Part model, mm, in its own coordinate system. Round coordinates to 2 decimals unless told otherwise and drop trailing zeros. Order: outer loops, then holes, each group sorted by start corner. A loop starts at its lowest first (then second) coordinate and runs counter-clockwise, first axis right, second up. Notation, with made-up numbers: M -15.75,-10.75 L 36.25,-10.75 A24 ccw 36.25,5.25 Z; hole C -40,48 d1. An arc over 180 degrees is marked long. Write each question's results on one line, items separated by ' | '. Start each with the question number.
1. Probe L1, parallel to Y at x = 1.15, z = -12.7; L2, parallel to Y at x = 2.05, z = -45; L3, parallel to Z at x = 2.3, y = -13.5. List the from-to ranges inside material, lowest first. Write a range as [from, to].
2. Drop a flat-ended pin along its axis: pin 1 Ø1.5 at (x, y) = (0.5, -61) entering from +Z. Give the stop position or say it passes through.
3. Band-saw the part on D-D, the plane z = -68.5. List the corners of the cut face in (x, y) (3 decimals).
4. Band-saw the part on A-A, the plane z = -50.8. List the corners of the cut face in (x, y) (3 decimals), then the cut area to 3 significant figures.
5. Band-saw the part on B-B, the plane x = 1.4. Give the number of separate pieces and of enclosed holes in the cut face, then the cut area to 3 significant figures.
6. Band-saw the part on C-C, the plane y = -12.7. List the corners of the cut face in (x, z) (3 decimals), then the cut area to 3 significant figures.
Autodesk Inventor part; units mm, degrees
ref_plane "YZ Plane" through (0, 0, 0) normal (1, 0, 0) x (0, 1, 0)
ref_plane "XZ Plane" through (0, 0, 0) normal (0, 1, 0) x (-1, 0, 0)
ref_plane "XY Plane" through (0, 0, 0) normal (0, 0, 1) x (1, 0, 0)
sketch "Sketch1" plane through (0, 0, 0) normal (1, 0, 0) x (0, 1, 0)
  line L0 (0, 0) -> (0, -101.6)
  line L1 (0, -101.6) -> (-52.8555, -156.4884)
  line L2 (-25.4, 2.4125) -> (-25.4, -91.3586)
  line L3 (-25.4, -91.3586) -> (-71.1516, -138.8699)
  line L4 (-52.8555, -156.4884) -> (-71.1516, -138.8699)
  line L5 (0, 0) -> (-25.4, 0)
  dimension "d0" = 101.6
  dimension "d1" = 25.4
  dimension "d2" = 25.4
  dimension "d3" = 76.2
  dimension "d4" = 136.081
extrude "Extrusion1" add sketch "Sketch1" along normal blind 3.175
sketch "Sketch2" plane through (0, 0, 0) normal (-1, 0, 0) x (0, 0, 1)
  circle A0 centre (-12.7, -12.7) radius 3.3734
  circle A1 centre (-31.75, -12.7) radius 3.3734
  circle A2 centre (-50.8, -12.7) radius 3.3734
  line L0 (0, -25.4) -> (0, 0)
  line L1 (0, -12.7) -> (-114.7885, -12.7) construction
  line L2 (-156.4884, -52.8555) -> (-101.6, 0)
  circle A3 centre (-138.5311, -53.1943) radius 3.3734
  circle A4 centre (-120.235, -35.5758) radius 3.3734
  circle A5 centre (-101.9388, -17.9573) radius 3.3734
  line L3 (-91.3586, -25.4) -> (-138.8699, -71.1516)
  line L4 (-156.4884, -52.8555) -> (-138.8699, -71.1516)
  dimension "d7" = 6.7469
  dimension "d8" = 6.7469
  dimension "d9" = 6.7469
  dimension "d10" = 12.7
  dimension "d11" = 19.05
  dimension "d12" = 19.05
  dimension "d15" = 6.7469
  dimension "d16" = 6.7469
  dimension "d17" = 6.7469
  dimension "d18" = 12.7
  dimension "d19" = 12.7
  dimension "d20" = 12.7
  dimension "d21" = 12.7
  dimension "d22" = 38.1
  dimension "d23" = 63.5
extrude "Extrusion2" cut sketch "Sketch2" against normal blind 3.175
properties part number "lower gusset" material "Aluminum 6061"
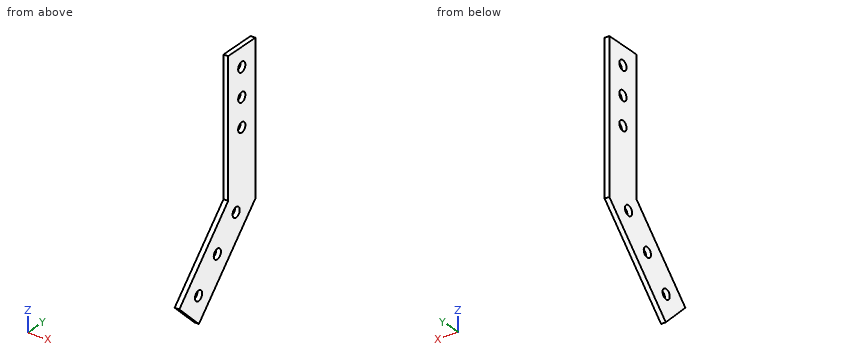
Solution:
1) L1: [-25.4, -16.07], [-9.33, 0] | L2: [-25.4, 0] | L3: [-115.62, -54.08], [-47.52, -35.03], [-28.47, -15.98], [-9.42, 0]
2) pin 1: z = -127.55
3) outline: M 0,-25.4 L 3.175,-25.4 L 3.175,0 L 0,0 Z
4) outline: M 0,-25.4 L 3.175,-25.4 L 3.175,-16.073 L 0,-16.073 Z; M 0,-9.327 L 3.175,-9.327 L 3.175,0 L 0,0 Z | area: 59.2 mm^2
5) separate pieces: 1 | enclosed holes: 6 | area: 4,040 mm^2
6) outline: M 0,-114.788 L 3.175,-114.788 L 3.175,-54.173 L 0,-54.173 Z; M 0,-47.427 L 3.175,-47.427 L 3.175,-35.123 L 0,-35.123 Z; M 0,-28.377 L 3.175,-28.377 L 3.175,-16.073 L 0,-16.073 Z; M 0,-9.327 L 3.175,-9.327 L 3.175,0 L 0,0 Z | area: 300 mm^2
